Design review of the part built by this model. Coordinates are the model's own, in mm. Face numbers are marked on the shaded views. A direction names the side the tool comes from. Coordinates: 2 decimals unless noted, no trailing zeros. Loops run counter-clockwise (first coordinate to the right, second up) from the corner with the lowest first, then second, coordinate; pieces in that order, holes last. Notation, with made-up numbers: (89.5, 8) -> (138.5, 8) arc R34 ccw to (138.5, 39) -> close; hole circle Ø6 at (47, 41). An arc over 180 degrees is marked (long way). Answer as a JSON object with one key per item and string values.
```python
from build123d import *

# Parameters (mm, degrees)
F1_DEPTH  = 25.4
F4_DEPTH  = 25.401
F3_R      = 6.35
F5_DEPTH  = 25.401
F8_DEPTH  = 12.701
F9_DEPTH  = 12.701
F11_DEPTH = 12.701


with BuildPart() as f1:
    # F0 (on Front) → F1 (new body)
    with BuildSketch(Plane.XZ):
        Polygon((-51.3122697964, 54.3005044411), (-76.7122697964, 54.3005044411), (-76.7122697964, 16.2005044411), (-6.8622697964, 16.2005044411), (-6.8622697964, 28.9005044411), (-51.3122697964, 28.9005044411), align=None)
    extrude(amount=F1_DEPTH)

    # F2 (on face) → F4 (cut, through all)
    with BuildSketch(Plane.XZ.offset(25.4)):
        with BuildLine():
            ThreePointArc((-76.7122697964, 41.6005044411), (-72.9925259175, 50.5807605622), (-64.0122697964, 54.3005044411))
            Line((-64.0122697964, 54.3005044411), (-76.7122697964, 54.3005044411))
            Line((-76.7122697964, 54.3005044411), (-76.7122697964, 41.6005044411))
        make_face()
        with BuildLine():
            ThreePointArc((-64.0122697964, 54.3005044411), (-55.0320136754, 50.5807605622), (-51.3122697964, 41.6005044411))
            Line((-51.3122697964, 41.6005044411), (-51.3122697964, 54.3005044411))
            Line((-51.3122697964, 54.3005044411), (-64.0122697964, 54.3005044411))
        make_face()
    extrude(amount=-F4_DEPTH, mode=Mode.SUBTRACT)

    # F3 (on face) → F5 (cut, through all)
    with BuildSketch(Plane.XZ.offset(25.4)):
        with Locations((-64.0122697964, 41.6005044411)):
            Circle(F3_R)
    extrude(amount=-F5_DEPTH, mode=Mode.SUBTRACT)

    # F6 (on face) → F8 (cut, through all)
    with BuildSketch(Plane.XY.offset(28.9005044411)):
        with BuildLine():
            ThreePointArc((-38.6122697964, -19.05), (-34.1221417359, -17.1901280605), (-32.2622697964, -12.7))
            ThreePointArc((-32.2622697964, -12.7), (-34.1221417359, -8.2098719395), (-38.6122697964, -6.35))
            ThreePointArc((-38.6122697964, -6.35), (-44.9622697964, -12.7), (-38.6122697964, -19.05))
        make_face()
        with BuildLine():
            ThreePointArc((-13.2122697964, -12.7), (-15.0721417359, -8.2098719395), (-19.5622697964, -6.35))
            ThreePointArc((-19.5622697964, -6.35), (-25.9122697964, -12.7), (-19.5622697964, -19.05))
            ThreePointArc((-19.5622697964, -19.05), (-15.0721417359, -17.1901280605), (-13.2122697964, -12.7))
        make_face()
    extrude(amount=-F8_DEPTH, mode=Mode.SUBTRACT)

    # F7 (on face) → F9 (cut, through all)
    with BuildSketch(Plane.XY.offset(28.9005044411)):
        with BuildLine():
            Line((-21.0363403239, -6.5234624522), (-37.1381992689, -6.5234624522))
            ThreePointArc((-37.1381992689, -6.5234624522), (-33.6281526304, -8.7654001379), (-32.2622697964, -12.7))
            ThreePointArc((-32.2622697964, -12.7), (-34.1221417359, -17.1901280605), (-38.6122697964, -19.05))
            Line((-38.6122697964, -19.05), (-19.5622697964, -19.05))
            ThreePointArc((-19.5622697964, -19.05), (-25.8687550865, -13.4421208026), (-21.0363403239, -6.5234624522))
        make_face()
    extrude(amount=-F9_DEPTH, mode=Mode.SUBTRACT)

    # F10 (on face) → F11 (cut, through all)
    with BuildSketch(Plane.XY.offset(28.9005044411)):
        with BuildLine():
            ThreePointArc((-19.5622697964, 0), (-10.5820136754, -3.7197438789), (-6.8622697964, -12.7))
            Line((-6.8622697964, -12.7), (-6.8622697964, 0))
            Line((-6.8622697964, 0), (-19.5622697964, 0))
        make_face()
        with BuildLine():
            Line((-6.8622697964, -25.4), (-6.8622697964, -12.7))
            ThreePointArc((-6.8622697964, -12.7), (-10.5820136754, -21.6802561211), (-19.5622697964, -25.4))
            Line((-19.5622697964, -25.4), (-6.8622697964, -25.4))
        make_face()
    extrude(amount=-F11_DEPTH, mode=Mode.SUBTRACT)


solid = f1.part
```
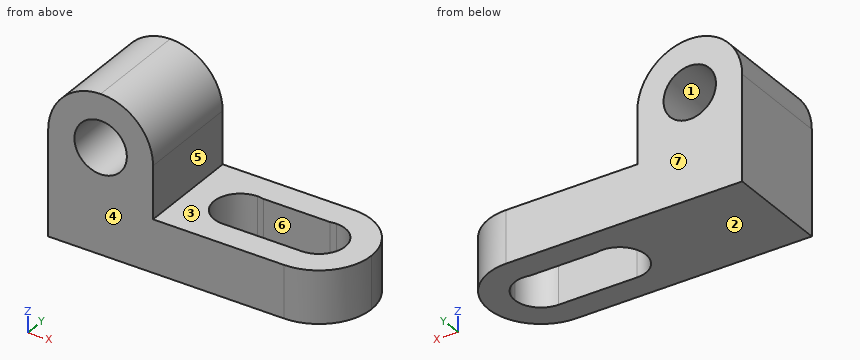
1) Add section D-D, the plane z = 36.5. Give the boundary of the cut face in (x, y).
Completed:
{"outline": "(-76.71, -25.4) -> (-67.79, -25.4) -> (-67.79, 0) -> (-76.71, 0) -> close; (-60.23, -25.4) -> (-51.31, -25.4) -> (-51.31, 0) -> (-60.23, 0) -> close"}
2) Add section C-C, the plane y = -24. Give the boundary of the cut face in (x, z), and give its area (3 significant figures).
Completed:
{"outline": "(-76.71, 16.2) -> (-13.77, 16.2) -> (-13.77, 28.9) -> (-51.31, 28.9) -> (-51.31, 41.6) arc R12.7 ccw to (-76.71, 41.6) -> close; hole circle Ø12.7 at (-64.01, 41.6)", "area": "1,250 mm²"}
3) Add section A-A, the plane x = -35. Give the boundary of the cut face in (y, z), and give its area (3 significant figures).
Completed:
{"outline": "(-25.4, 16.2) -> (-19.05, 16.2) -> (-19.05, 28.9) -> (-25.4, 28.9) -> close; (-6.52, 16.2) -> (0, 16.2) -> (0, 28.9) -> (-6.52, 28.9) -> close", "area": "163 mm²"}
4) The part is to be moulded in two halves that separate along Z. For the marked faces 1, 2, 3 and 4, say which applies: pulls with the +Z half, pulls with the -Z half, needs draft (parallel to the pull), parting line crosses it, or undercut.
Completed:
{"face 1": "undercut", "face 2": "pulls with the -Z half", "face 3": "pulls with the +Z half", "face 4": "needs draft"}
5) Wall thickness on probe 1 along Y at (x, z) = (-30, 20); probe 2 along X at (y, z) = (-12.25, 18.5); probe 3 along X at (y, z) = (-7.5, 22.5): over which ranges is each line inside the solid? List them lowest first.
Completed:
{"probe 1": "-25.4 to -19.05, -6.52 to 0", "probe 2": "-76.71 to -44.95, -13.23 to -6.87", "probe 3": "-76.71 to -42.26, -15.92 to -7.98"}
6) For the marked faces 5, 6 and 7, list the 3-axis set-ups (+Z, -Z, +X, -X, +Y, -Y) from which the entire face can be reached by the end or side of a thin tool; tool diameter is ignored.
Completed:
{"face 5": "+Z, +X, +Y, -Y", "face 6": "+Z, -Z", "face 7": "+Z, -Z, +X, -X, +Y"}
7) Clearance check with flat-ended pins moving along their axes: pin 1 Ø1.5 at (x, y) = (-62, -8) entering from +Z; pin 2 Ø16.5 at (x, z) = (-64.01, 41.6) entering from +Y; pin 3 Ø1.5 at (x, y) = (-60, -19.5) entering from +Z; pin 4 Ø12 at (y, z) = (-21.5, 50) entering from +X. State where each tip first meets the part, or that it passes through.
Completed:
{"pin 1": "z = 54.24", "pin 2": "y = 0", "pin 3": "z = 53.87", "pin 4": "x = -51.54"}
8) Add section B-B, the plane z = 28. Give the boundary of the cut face in (x, y), and give its area (3 significant figures).
Completed:
{"outline": "(-76.71, -25.4) -> (-19.56, -25.4) arc R12.7 ccw to (-19.56, 0) -> (-76.71, 0) -> close; hole (-38.61, -19.05) -> (-19.56, -19.05) arc R6.35 ccw (long way) to (-21.04, -6.52) -> (-37.14, -6.52) arc R6.35 ccw (long way) to start", "area": "1,340 mm²"}
